from build123d import *

# Parameters (mm, degrees)
SKETCH_W        = 85
SKETCH_H        = 85
PAD_DEPTH       = 3
SKETCH001_W     = 25
SKETCH001_H     = 25
POCKET_DEPTH    = 5
CHAMFER_SIZE    = 1
SKETCH002_R     = 2
POCKET001_DEPTH = 1.5


with BuildPart() as part:
    # Sketch → Pad (new body)
    with BuildSketch(Plane.XY):
        Rectangle(SKETCH_W, SKETCH_H)
    extrude(amount=PAD_DEPTH)

    # Sketch001 (on Face6 of Pad) → Pocket (cut)
    with BuildSketch(Plane.XY.offset(3)):
        Rectangle(SKETCH001_W, SKETCH001_H)
    extrude(amount=-POCKET_DEPTH, mode=Mode.SUBTRACT)

    # Chamfer
    chamfer_edges = [part.edges().sort_by_distance(p)[0] for p in [
        (42.5, 0, 3),
        (0, -42.5, 3),
        (-42.5, 0, 3),
        (0, 42.5, 3),
    ]]
    chamfer(chamfer_edges, length=CHAMFER_SIZE)

    # Sketch002 (on Face8 of Chamfer) → Pocket001 (cut)
    with BuildSketch(Plane.XY.offset(3)):
        with Locations((-17.5, 17.5)):
            Circle(SKETCH002_R)
        with Locations((-17.5, -17.5)):
            Circle(SKETCH002_R)
        with Locations((17.5, -17.5)):
            Circle(SKETCH002_R)
        with Locations((17.5, 17.5)):
            Circle(SKETCH002_R)
    extrude(amount=-POCKET001_DEPTH, mode=Mode.SUBTRACT)


solid = part.part
Part model, mm, in its own coordinate system. A direction names the side the tool comes from. Coordinates: 2 decimals unless noted, no trailing zeros. Write each loop counter-clockwise with the first axis right and the second up, starting at its lowest first coordinate (ties: lowest second). Pieces come first, ordered by that corner, then holes. Notation, with made-up numbers: M -21.75,-35 L 18.25,-35 A29 ccw 18.25,-15 Z; hole C 63.25,54 d11. An arc over 180 degrees is marked long. Return JSON: item names as keys, results as strings.
1. Probe L1, parallel to Y at x = 12, z = 1.25; L2, parallel to Y at x = -17.5, z = 2.55; L3, parallel to Y at x = -17.5, z = 2.3. List the from-to ranges inside material, lowest first.
Determined:
{"L1": "-42.5 to -12.5, 12.5 to 42.5", "L2": "-41.95 to -19.5, -15.5 to 15.5, 19.5 to 41.95", "L3": "-42.2 to -19.5, -15.5 to 15.5, 19.5 to 42.2"}
2. Pull direction X, two halves, no side cores. Call faces 1 (the face through (-19, 1, 0)), 2 (the face through (0, 12.5, 2)), 3 (the face through (42.5, -1, 1)), 4 (the face through (-42.5, -1, 1)): pulls with the +X half, pulls with the -X half, needs draft (parallel to the pull), parting line crosses it, or undercut.
Determined:
{"face 1": "needs draft", "face 2": "undercut", "face 3": "pulls with the +X half", "face 4": "pulls with the -X half"}
3. Saw through at A-A, the plane y = 11. Write the cut outline in (x, z).
Determined:
{"outline": "M -42.5,0 L -12.5,0 L -12.5,3 L -41.5,3 L -42.5,2 Z; M 12.5,0 L 42.5,0 L 42.5,2 L 41.5,3 L 12.5,3 Z"}
4. Saw through at D-D, the plane x = 17.5. Write the cut outline in (y, z), then the cut area to 3 significant figures.
Determined:
{"outline": "M -42.5,0 L 42.5,0 L 42.5,2 L 41.5,3 L 19.5,3 L 19.5,1.5 L 15.5,1.5 L 15.5,3 L -15.5,3 L -15.5,1.5 L -19.5,1.5 L -19.5,3 L -41.5,3 L -42.5,2 Z", "area": "242 mm²"}
5. Saw through at C-C, the plane z = 1. Write the cut outline in (x, y), then the cut area to 3 significant figures.
Determined:
{"outline": "M -42.5,-42.5 L 42.5,-42.5 L 42.5,42.5 L -42.5,42.5 Z; hole M -12.5,-12.5 L 12.5,-12.5 L 12.5,12.5 L -12.5,12.5 Z", "area": "6,600 mm²"}
6. Flat gauge pin, fed straight in: pin 1 Ø1.2 at (x, y) = (17, -18) entering from +Z. Where does the tip first touch, or does it go through?
Determined:
{"pin 1": "z = 1.5"}
7. 3-axis set-ups, long thin cutter, end or side, ignore diameter. For faces 5 (the face through (-1, -42.5, 1)), 6 (the face through (17.24, 19.483, 2.26)), 7 (the face through (-12.5, 0, 2)): which of +Z, -Z, +X, -X, +Y, -Y reach the whole face in a straight line?
Determined:
{"face 5": "+Z, -Z, +X, -X, -Y", "face 6": "+Z", "face 7": "+Z, -Z"}
